```python
from build123d import *

# Parameters (mm, degrees)
Y_KSEKLIK_EKSTR_ZYON1_DEPTH      = 10
Y_KSEKLIK_EKSTR_ZYON2_DEPTH      = 10
Y_KSEKLIK_EKSTR_ZYON2_DEPTH_BACK = 10
IZIM3_W                          = 15.866666667
IZIM3_H                          = 5
IZIM5_R                          = 1.7
KES_EKSTR_ZYON1_DEPTH            = 36
IZIM9_R                          = 1.7
KES_EKSTR_ZYON2_DEPTH            = 36


with BuildPart() as part:
    # Çizim2 → Yükseklik-Ekstrüzyon1 (new body)
    with BuildSketch(Plane.XY):
        Polygon((0, 0), (0, 79.333333333), (0, 85), (2.833333333, 85), (2.833333333, 68), (13.033333333, 68), (13.033333333, 85), (15.866666667, 85), (15.866666667, 79.333333333), (15.866666667, 0), align=None)
    extrude(amount=Y_KSEKLIK_EKSTR_ZYON1_DEPTH)

    # Çizim3 → Yükseklik-Ekstrüzyon2 (add, two sides: drawn at the far end of the back side and taken through both)
    with BuildSketch(Plane(origin=(0, 0, 0), x_dir=(-1, 0, 0), z_dir=(0, 0, -1)).offset(-Y_KSEKLIK_EKSTR_ZYON2_DEPTH_BACK)):
        with Locations((-7.933333334, -2.5)):
            Rectangle(IZIM3_W, IZIM3_H)
    extrude(amount=Y_KSEKLIK_EKSTR_ZYON2_DEPTH + Y_KSEKLIK_EKSTR_ZYON2_DEPTH_BACK)

    # Çizim5 → Kes-Ekstrüzyon1 (cut)
    with BuildSketch(Plane(origin=(15.866666667, 0, 0), x_dir=(0, 0, -1), z_dir=(1, 0, 0))):
        with Locations((-5, 81)):
            Circle(IZIM5_R)
    extrude(amount=-KES_EKSTR_ZYON1_DEPTH, mode=Mode.SUBTRACT)

    # Çizim9 → Kes-Ekstrüzyon2 (cut)
    with BuildSketch(Plane(origin=(0, 0, 0), x_dir=(1, 0, 0), z_dir=(0, 1, 0))):
        with Locations(Location((7.933333333, 5, 0), (0, 0, 270))):
            Circle(IZIM9_R)
    extrude(amount=-KES_EKSTR_ZYON2_DEPTH, mode=Mode.SUBTRACT)


solid = part.part
```
Source: CAD feature listing. Evaluate the final solid. Frame: model axes, mm. A direction names the side the tool comes from. Round coordinates to 2 decimals unless told otherwise and drop trailing zeros. Write each loop counter-clockwise with the first axis right and the second up, starting at its lowest first coordinate (ties: lowest second). Pieces come first, ordered by that corner, then holes. Notation, with made-up numbers: M 89,-35.75 L 118,-35.75 A23 ccw 118,-6.75 Z; hole C -36.5,-13.5 d9. An arc over 180 degrees is marked long. Answer as a JSON object with one key per item and string values. Group by question number.
(1) Section query C-C on y = 81. Output: boundary loops of the cut face in (x, z), then the cut area to 3 significant figures.
(2) Reachability of faces 1 (the flat face through (15.867, 39, 5)), 2 (the flat face through (8, 43, 0)), 3 (the flat face through (13.033, 76, 5)) from +Z, -Z, +X, -X, +Y, -Y: full face, straight path, thin tool, end or side. Return the list, or none.
(3) Mould query, pull axis X, two halves, no side actions, for faces 4 (the flat face through (2.833, 77, 5)), 5 (the cylindrical face through (9.62, -2.46, -5.22)), 6 (the flat face through (8, -5, 0)), 7 (the flat face through (0, 39, 5)). Classes: +X half, -X half, draft (parallel to the pull), parting line (faces both ways), or undercut.
(4) Section query D-D on x = 7. Output: boundary loops of the cut face in (y, z).
(5) Ray query, line 1 (Z direction, x = 0.85, y = 81); line 2 (Z direction, x = 9, y = 55.5); line 3 (Y direction, x = 11.25, z = -4.5). Return the intervals inside material, ascending. Write a range as [from, to].
(6) Section query B-B on x = 2. Output: boundary loops of the cut face in (y, z), then the cut area to 3 significant figures.
(7) Section query A-A on z = -5. Output: boundary loops of the cut face in (x, y).
(8) First-contact query: pin 1 (2 mm diameter, centred on y = 81, z = 5, fed in from +X); pin 2 (3 mm diameter, centred on x = 8, z = 5.5, fed in from +Y); pin 3 (5 mm diameter, centred on x = 9, y = 58.5, fed in from -Z); pin 4 (3 mm diameter, centred on x = 14, z = -2, fed in from +Y). Flat tips, straight axial feed; report the tip coordinate or a pass-through.
Computed values:
{
 "1": {"outline": "M 0,0 L 2.83,0 L 2.83,3.3 L 0,3.3 Z; M 0,6.7 L 2.83,6.7 L 2.83,10 L 0,10 Z; M 13.03,0 L 15.87,0 L 15.87,3.3 L 13.03,3.3 Z; M 13.03,6.7 L 15.87,6.7 L 15.87,10 L 13.03,10 Z", "area": "37.4 mm^2"},
 "2": {"face 1": "+Z, -Z, +X, +Y, -Y", "face 2": "-Z, +X, -X, +Y", "face 3": "+Z, -Z, +Y"},
 "3": {"face 4": "undercut", "face 5": "undercut", "face 6": "draft", "face 7": "-X half"},
 "4": {"outline": "M -5,-10 L 0,-10 L 0,-6.42 L -5,-6.42 Z; M -5,-3.58 L 0,-3.58 L 0,0 L 68,0 L 68,10 L -5,10 Z"},
 "5": {"line 1": "[0, 3.3], [6.7, 10]", "line 2": "[0, 10]", "line 3": "[-5, 0]"},
 "6": {"outline": "M -5,-10 L 0,-10 L 0,0 L 85,0 L 85,10 L -5,10 Z; hole C 81,5 d3.4", "area": "941 mm^2"},
 "7": {"outline": "M 0,-5 L 6.23,-5 L 6.23,0 L 0,0 Z; M 9.63,-5 L 15.87,-5 L 15.87,0 L 9.63,0 Z"},
 "8": {"pin 1": "through", "pin 2": "y = 68", "pin 3": "z = 0", "pin 4": "y = 0"}
}
